Read the model definition and answer for the solid it produces. Units are mm, in the model's axes. Coordinates: 2 decimals unless noted, no trailing zeros. Write each loop counter-clockwise with the first axis right and the second up, starting at its lowest first coordinate (ties: lowest second). Pieces come first, ordered by that corner, then holes. Notation, with made-up numbers: (-21, 74.5) -> (-5, 74.5) arc R20 cw to (-5, 108.5) -> close; hole circle Ø5 at (86, -1). An arc over 180 degrees is marked (long way). Answer in a Markdown table with one row per item. Add a question column.
Item 1: Section C-C on z = 1.9 is taken. Count the separate pieces of the cut face and the enclosed holes in it, then the cut area to 3 significant figures.
Item 2: Given pin 1 Ø4 at (x, y) = (101.6, -72.39) entering from +Z, flat-ended and moving along its own axis, determine where the tip first touches the part or whether it passes through.
Item 3: Section A-A on y = 17 is taken. Write down the section's boundary in (x, z) (3 decimals).
Item 4: Section B-B on x = 40 is taken. Write down the section's boundary in (y, z) (3 decimals), then the cut area to 3 significant figures.
Item 5: Straight lines are drawn through the part: line 1 (X direction, y = -42, z = 2.3); line 2 (Y direction, x = 36.5, z = 0.65) (3 decimals); line 3 (X direction, y = 139.7, z = 2.1). For each, find the intervals that lie inside material, in ascending order. Write a range as from..to.
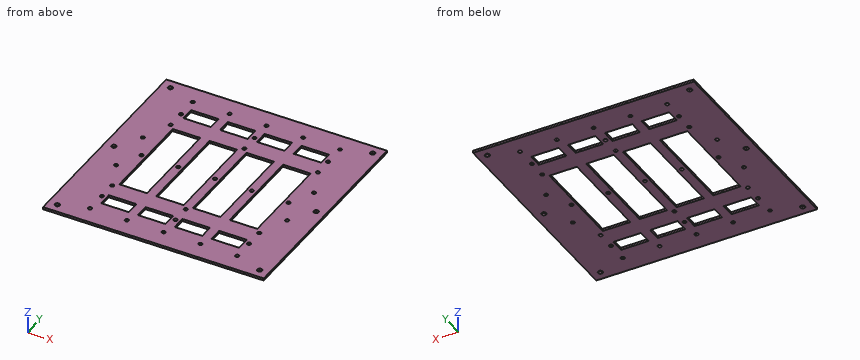
```python
from build123d import *

# Parameters (mm, degrees)
SKETCH1_W           = 304.8
SKETCH1_H           = 304.8
SKETCH1_R           = 2.54
SKETCH1_R_2         = 3.2639
SKETCH1_W_2         = 38.1
SKETCH1_H_2         = 132.08
SKETCH1_H_3         = 19.05
BOSS_EXTRUDE1_DEPTH = 3.175


with BuildPart() as part:
    # Sketch1 → Boss-Extrude1 (new body)
    with BuildSketch(Plane.XY):
        Rectangle(SKETCH1_W, SKETCH1_H)
        with Locations((-101.6, 0)):
            Circle(SKETCH1_R, mode=Mode.SUBTRACT)
        with Locations((-50.8, 0)):
            Circle(SKETCH1_R, mode=Mode.SUBTRACT)
        Circle(SKETCH1_R, mode=Mode.SUBTRACT)
        with Locations((101.6, 0)):
            Circle(SKETCH1_R, mode=Mode.SUBTRACT)
        with Locations((50.8, 0)):
            Circle(SKETCH1_R, mode=Mode.SUBTRACT)
        with Locations((-50.8, 127)):
            Circle(SKETCH1_R, mode=Mode.SUBTRACT)
        with Locations((0, 127)):
            Circle(SKETCH1_R, mode=Mode.SUBTRACT)
        with Locations((50.8, 127)):
            Circle(SKETCH1_R, mode=Mode.SUBTRACT)
        with Locations((-101.6, 72.39)):
            Circle(SKETCH1_R, mode=Mode.SUBTRACT)
        with Locations((0, 72.39)):
            Circle(SKETCH1_R, mode=Mode.SUBTRACT)
        with Locations((101.6, 72.39)):
            Circle(SKETCH1_R, mode=Mode.SUBTRACT)
        with Locations((-101.6, -72.39)):
            Circle(SKETCH1_R, mode=Mode.SUBTRACT)
        with Locations((0, -72.39)):
            Circle(SKETCH1_R, mode=Mode.SUBTRACT)
        with Locations((101.6, -72.39)):
            Circle(SKETCH1_R, mode=Mode.SUBTRACT)
        with Locations((50.8, -127)):
            Circle(SKETCH1_R, mode=Mode.SUBTRACT)
        with Locations((0, -127)):
            Circle(SKETCH1_R, mode=Mode.SUBTRACT)
        with Locations((-50.8, -127)):
            Circle(SKETCH1_R, mode=Mode.SUBTRACT)
        with Locations((-101.6, 97.79)):
            Circle(SKETCH1_R, mode=Mode.SUBTRACT)
        with Locations((0, 97.79)):
            Circle(SKETCH1_R, mode=Mode.SUBTRACT)
        with Locations((101.6, 97.79)):
            Circle(SKETCH1_R, mode=Mode.SUBTRACT)
        with Locations((101.6, 127)):
            Circle(SKETCH1_R, mode=Mode.SUBTRACT)
        with Locations((-101.6, 127)):
            Circle(SKETCH1_R, mode=Mode.SUBTRACT)
        with Locations((-118.11, 33.02)):
            Circle(SKETCH1_R, mode=Mode.SUBTRACT)
        with Locations((-101.6, -127)):
            Circle(SKETCH1_R, mode=Mode.SUBTRACT)
        with Locations((101.6, -127)):
            Circle(SKETCH1_R, mode=Mode.SUBTRACT)
        with Locations((101.6, -97.79)):
            Circle(SKETCH1_R, mode=Mode.SUBTRACT)
        with Locations((0, -97.79)):
            Circle(SKETCH1_R, mode=Mode.SUBTRACT)
        with Locations((-101.6, -97.79)):
            Circle(SKETCH1_R, mode=Mode.SUBTRACT)
        with Locations((-118.11, -33.02)):
            Circle(SKETCH1_R, mode=Mode.SUBTRACT)
        with Locations((-139.7, 139.7)):
            Circle(SKETCH1_R_2, mode=Mode.SUBTRACT)
        with Locations((-139.7, 0)):
            Circle(SKETCH1_R_2, mode=Mode.SUBTRACT)
        with Locations((-139.7, -139.7)):
            Circle(SKETCH1_R_2, mode=Mode.SUBTRACT)
        with Locations((139.7, -139.7)):
            Circle(SKETCH1_R_2, mode=Mode.SUBTRACT)
        with Locations((139.7, 0)):
            Circle(SKETCH1_R_2, mode=Mode.SUBTRACT)
        with Locations((139.7, 139.7)):
            Circle(SKETCH1_R_2, mode=Mode.SUBTRACT)
        with Locations((118.11, -33.02)):
            Circle(SKETCH1_R, mode=Mode.SUBTRACT)
        with Locations((118.11, 33.02)):
            Circle(SKETCH1_R, mode=Mode.SUBTRACT)
        with Locations((-76.2, 0)):
            Rectangle(SKETCH1_W_2, SKETCH1_H_2, mode=Mode.SUBTRACT)
        with Locations((-25.4, 0)):
            Rectangle(SKETCH1_W_2, SKETCH1_H_2, mode=Mode.SUBTRACT)
        with Locations((25.4, 0)):
            Rectangle(SKETCH1_W_2, SKETCH1_H_2, mode=Mode.SUBTRACT)
        with Locations((76.2, 0)):
            Rectangle(SKETCH1_W_2, SKETCH1_H_2, mode=Mode.SUBTRACT)
        with Locations((-25.4, 101.6)):
            Rectangle(SKETCH1_W_2, SKETCH1_H_3, mode=Mode.SUBTRACT)
        with Locations((-76.2, 101.6)):
            Rectangle(SKETCH1_W_2, SKETCH1_H_3, mode=Mode.SUBTRACT)
        with Locations((76.2, 101.6)):
            Rectangle(SKETCH1_W_2, SKETCH1_H_3, mode=Mode.SUBTRACT)
        with Locations((25.4, 101.6)):
            Rectangle(SKETCH1_W_2, SKETCH1_H_3, mode=Mode.SUBTRACT)
        with Locations((-76.2, -101.6)):
            Rectangle(SKETCH1_W_2, SKETCH1_H_3, mode=Mode.SUBTRACT)
        with Locations((-25.4, -101.6)):
            Rectangle(SKETCH1_W_2, SKETCH1_H_3, mode=Mode.SUBTRACT)
        with Locations((25.4, -101.6)):
            Rectangle(SKETCH1_W_2, SKETCH1_H_3, mode=Mode.SUBTRACT)
        with Locations((76.2, -101.6)):
            Rectangle(SKETCH1_W_2, SKETCH1_H_3, mode=Mode.SUBTRACT)
    extrude(amount=BOSS_EXTRUDE1_DEPTH)


solid = part.part
```
Results below:
| question | item | result |
|---|---|---|
| 1 | separate pieces | 1 |
| 1 | enclosed holes | 49 |
| 1 | area | 66,100 mm2 |
| 2 | pin 1 | passes through |
| 3 | outline | (-152.4, 0) -> (-95.25, 0) -> (-95.25, 3.175) -> (-152.4, 3.175) -> close; (-57.15, 0) -> (-44.45, 0) -> (-44.45, 3.175) -> (-57.15, 3.175) -> close; (-6.35, 0) -> (6.35, 0) -> (6.35, 3.175) -> (-6.35, 3.175) -> close; (44.45, 0) -> (57.15, 0) -> (57.15, 3.175) -> (44.45, 3.175) -> close; (95.25, 0) -> (152.4, 0) -> (152.4, 3.175) -> (95.25, 3.175) -> close |
| 4 | outline | (-152.4, 0) -> (-111.125, 0) -> (-111.125, 3.175) -> (-152.4, 3.175) -> close; (-92.075, 0) -> (-66.04, 0) -> (-66.04, 3.175) -> (-92.075, 3.175) -> close; (66.04, 0) -> (92.075, 0) -> (92.075, 3.175) -> (66.04, 3.175) -> close; (111.125, 0) -> (152.4, 0) -> (152.4, 3.175) -> (111.125, 3.175) -> close |
| 4 | area | 427 mm2 |
| 5 | line 1 | x = -152.4..-95.25, -57.15..-44.45, -6.35..6.35, 44.45..57.15, 95.25..152.4 |
| 5 | line 2 | y = -152.4..-111.125, -92.075..-66.04, 66.04..92.075, 111.125..152.4 |
| 5 | line 3 | x = -152.4..-142.96, -136.44..136.44, 142.96..152.4 |
